The figure shows three views and two pictorial views of one solid part (mm, origin at its lowest corner). Answer the questions. A direction names the side the tool comes from. Round coordinates to 2 decimals unless told otherwise and drop trailing zeros. Loops run counter-clockwise (first coordinate to the right, second up) from the corner with the lowest first, then second, coordinate; pieces in that order, holes last. Notation, with made-up numbers: (87, 31) -> (99, 31) arc R21 cw to (99, 41) -> close; hole circle Ø2 at (24, -28). An arc over 180 degrees is marked (long way). Use a Markdown table: item, result. Add a question column.
Q1. Which of the six approach directions +Z, -Z, +X, -X, +Y, -Y give full straight-line access (tool end or side, diameter ignored) to the marked faces 5, 6, 7, 8 and 9?
Q2. Section A-A on y = 12.5 is taken. Give the vertices of the cut face in (x, z), then the cut area to 3 significant figures.
Q3. For a pull along X with two mould halves and no side action, classify the marked faces 1, 2, 3 and 4 as released by +X, released by -X, zero draft, split by the parting line, or undercut.
Q4. Section D-D on x = 43.75 is taken. Give the vertices of the cut face in (y, z), then the cut area to 3 significant figures.
Q5. Consider line 1 (X direction, y = 1, z = 21.5); line 2 (X direction, y = 9.5, z = 17.5); line 3 (Y direction, x = 77, z = 14) (1 decimal). Determine where each line is inside the solid, lowest interval first.
Q6. Given pin 1 Ø3 at (x, y) = (10, 3) entering from -Z; pin 2 Ø4 at (y, z) = (8.5, 24) entering from -X; pin 3 Ø12.5 at (x, y) = (76, 12) entering from +Z; pin 4 Ø5 at (y, z) = (11, 12) entering from -X, each flat-ended and moving along its own axis, determine where each tip first touches the part or whether it passes through.
Q7. Section C-C on x = 75 is taken. Give the vertices of the cut face in (y, z).
Q8. Section B-B on y = 6 is taken. Give the vertices of the cut face in (x, z).
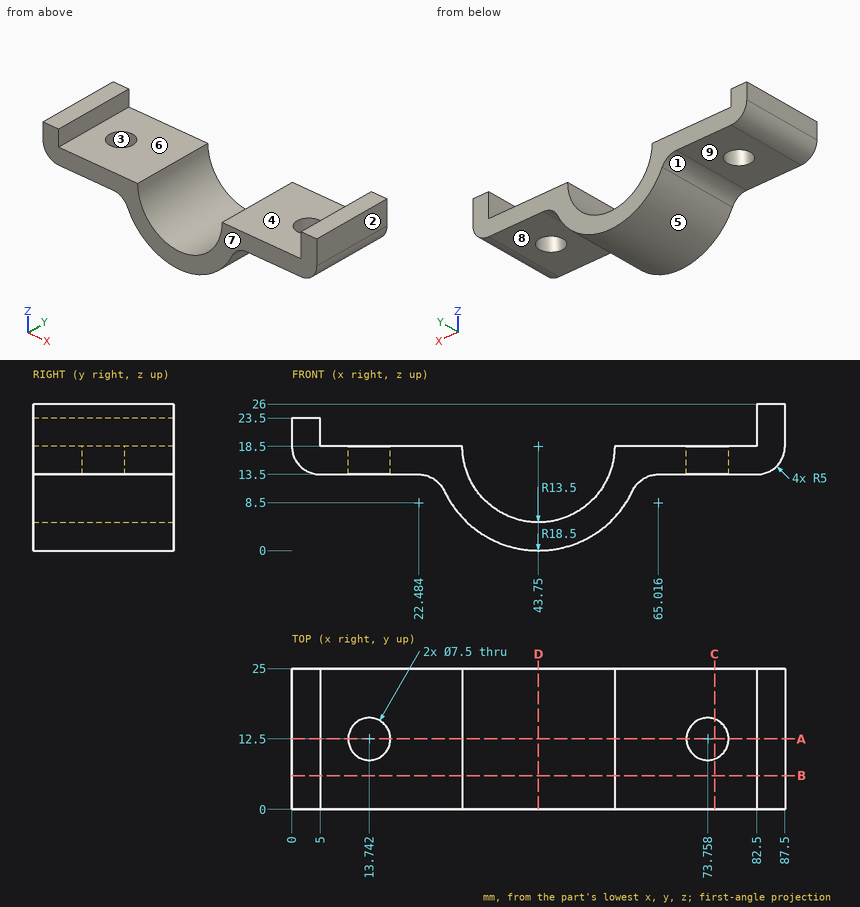
Checked values:
| question | item | result |
|---|---|---|
| 1 | face 5 | -Z, +Y, -Y |
| 1 | face 6 | +Z, +Y, -Y |
| 1 | face 7 | +Z, -Z, +X, -X, -Y |
| 1 | face 8 | -Z, +X, +Y, -Y |
| 1 | face 9 | -Z, -X, +Y, -Y |
| 2 | outline | (0, 18.5) arc R5 ccw to (5, 13.5) -> (9.99, 13.5) -> (9.99, 18.5) -> (5, 18.5) -> (5, 23.5) -> (0, 23.5) -> close; (17.49, 13.5) -> (22.48, 13.5) arc R5 cw to (27.01, 10.63) arc R18.5 ccw to (60.49, 10.63) arc R5 cw to (65.02, 13.5) -> (70.01, 13.5) -> (70.01, 18.5) -> (57.25, 18.5) arc R13.5 cw to (30.25, 18.5) -> (17.49, 18.5) -> close; (77.51, 13.5) -> (82.5, 13.5) arc R5 ccw to (87.5, 18.5) -> (87.5, 26) -> (82.5, 26) -> (82.5, 18.5) -> (77.51, 18.5) -> close |
| 2 | area | 487 mm2 |
| 3 | face 1 | released by -X |
| 3 | face 2 | released by +X |
| 3 | face 3 | undercut |
| 3 | face 4 | undercut |
| 4 | outline | (0, 0) -> (25, 0) -> (25, 5) -> (0, 5) -> close |
| 4 | area | 125 mm2 |
| 5 | line 1 | x = 0 to 5, 82.5 to 87.5 |
| 5 | line 2 | x = 0.1 to 11.49, 15.99 to 30.29, 57.21 to 71.51, 76.01 to 87.4 |
| 5 | line 3 | y = 0 to 10.6, 14.4 to 25 |
| 6 | pin 1 | stops at z = 13.5 |
| 6 | pin 2 | stops at x = 0 |
| 6 | pin 3 | stops at z = 18.5 |
| 6 | pin 4 | stops at x = 2 |
| 7 | outline | (0, 13.5) -> (8.96, 13.5) -> (8.96, 18.5) -> (0, 18.5) -> close; (16.04, 13.5) -> (25, 13.5) -> (25, 18.5) -> (16.04, 18.5) -> close |
| 8 | outline | (0, 18.5) arc R5 ccw to (5, 13.5) -> (22.48, 13.5) arc R5 cw to (27.01, 10.63) arc R18.5 ccw to (60.49, 10.63) arc R5 cw to (65.02, 13.5) -> (82.5, 13.5) arc R5 ccw to (87.5, 18.5) -> (87.5, 26) -> (82.5, 26) -> (82.5, 18.5) -> (57.25, 18.5) arc R13.5 cw to (30.25, 18.5) -> (5, 18.5) -> (5, 23.5) -> (0, 23.5) -> close |
